Work out the finished part from the listing and answer in its coordinate system (mm). A direction names the side the tool comes from. Round coordinates to 2 decimals unless told otherwise and drop trailing zeros. Loops run counter-clockwise (first coordinate to the right, second up) from the corner with the lowest first, then second, coordinate; pieces in that order, holes last.
```python
from build123d import *

# Parameters (mm, degrees)
BOSS_EXTRUDE1_DEPTH = 4
SKETCH10_R          = 4
SKETCH10_R_2        = 2.5
SKETCH10_W          = 20
SKETCH10_H          = 5
BOSS_EXTRUDE5_DEPTH = 5
SKETCH11_W          = 3
SKETCH11_H          = 50
SKETCH11_W_2        = 40
SKETCH11_H_2        = 3
BOSS_EXTRUDE6_DEPTH = 4
SKETCH12_R          = 2.5
CUT_EXTRUDE5_DEPTH  = 4
BOSS_EXTRUDE7_START = 2
SKETCH13_R          = 4
SKETCH13_R_2        = 2.5
BOSS_EXTRUDE7_DEPTH = 2
SKETCH14_R          = 2
CUT_EXTRUDE6_DEPTH  = 15
SKETCH15_R          = 3.5
CUT_EXTRUDE8_DEPTH  = 2
FILLET1_R           = 5


with BuildPart() as part:
    # Sketch1 → Boss-Extrude1 (new body)
    with BuildSketch(Plane(origin=(0, 0, 0), x_dir=(1, 0, 0), z_dir=(0, 1, 0))):
        Polygon((-68, 48), (-88, 28), (-88, -48), (88, -48), (88, 28), (68, 48), align=None)
    extrude(amount=BOSS_EXTRUDE1_DEPTH)

    # Sketch10 → Boss-Extrude5 (add)
    # profile 1 of 5: a face of its own
    with BuildSketch(Plane(origin=(0, 4, 0), x_dir=(1, 0, 0), z_dir=(0, 1, 0))):
        with Locations(Location((36.5, -38, 0), (0, 0, 270))):
            Circle(SKETCH10_R)
        with Locations(Location((36.5, -38, 0), (0, 0, 270))):
            Circle(SKETCH10_R_2, mode=Mode.SUBTRACT)
    # profile 2 of 5: a face of its own
    with BuildSketch(Plane(origin=(0, 4, 0), x_dir=(1, 0, 0), z_dir=(0, 1, 0))):
        with Locations(Location((-37.5, -37.5, 0), (0, 0, 270))):
            Circle(SKETCH10_R)
        with Locations(Location((-37.5, -37.5, 0), (0, 0, 270))):
            Circle(SKETCH10_R_2, mode=Mode.SUBTRACT)
    # profile 3 of 5: a face of its own
    with BuildSketch(Plane(origin=(0, 4, 0), x_dir=(1, 0, 0), z_dir=(0, 1, 0))):
        with Locations(Location((-35, 23, 0), (0, 0, 270))):
            Circle(SKETCH10_R)
        with Locations(Location((-35, 23, 0), (0, 0, 270))):
            Circle(SKETCH10_R_2, mode=Mode.SUBTRACT)
    # profile 4 of 5: a face of its own
    with BuildSketch(Plane(origin=(0, 4, 0), x_dir=(1, 0, 0), z_dir=(0, 1, 0))):
        with Locations((62, 26)):
            Rectangle(SKETCH10_W, SKETCH10_H)
    # profile 5 of 5: a face of its own
    with BuildSketch(Plane(origin=(0, 4, 0), x_dir=(1, 0, 0), z_dir=(0, 1, 0))):
        Polygon((42, 23), (42, 15), (39, 15), (39, 26), (44, 26), (44, 23), align=None)
    extrude(amount=BOSS_EXTRUDE5_DEPTH)

    # Sketch11 → Boss-Extrude6 (add)
    with BuildSketch(Plane(origin=(0, 4, 0), x_dir=(1, 0, 0), z_dir=(0, 1, 0))):
        Polygon((25, 43.5), (25, 45), (-25, 45), (-25, 43.5), (-25, 42), (25, 42), align=None)
        Polygon((-82, 20), (-83.5, 20), (-85, 20), (-85, -30), (-82, -30), align=None)
        with Locations((83.5, -5)):
            Rectangle(SKETCH11_W, SKETCH11_H)
        with Locations((-45, -43.5)):
            Rectangle(SKETCH11_W_2, SKETCH11_H_2)
    extrude(amount=BOSS_EXTRUDE6_DEPTH)

    # Sketch12 → Cut-Extrude5 (cut)
    with BuildSketch(Plane(origin=(0, 4, 0), x_dir=(1, 0, 0), z_dir=(0, 1, 0))):
        with Locations(Location((-63, 0, 0), (0, 0, 270))):
            Circle(SKETCH12_R)
        with Locations(Location((-33, 0, 0), (0, 0, 270))):
            Circle(SKETCH12_R)
        with Locations(Location((-3, 0, 0), (0, 0, 270))):
            Circle(SKETCH12_R)
    extrude(amount=-CUT_EXTRUDE5_DEPTH, mode=Mode.SUBTRACT)

    # Sketch13 → Boss-Extrude7 (add)
    # profile 1 of 3: a face of its own
    with BuildSketch(Plane(origin=(0, 4, 0), x_dir=(1, 0, 0), z_dir=(0, 1, 0)).offset(BOSS_EXTRUDE7_START)):
        with Locations(Location((-63, 0, 0), (0, 0, 270))):
            Circle(SKETCH13_R)
        with Locations(Location((-63, 0, 0), (0, 0, 270))):
            Circle(SKETCH13_R_2, mode=Mode.SUBTRACT)
    # profile 2 of 3: a face of its own
    with BuildSketch(Plane(origin=(0, 4, 0), x_dir=(1, 0, 0), z_dir=(0, 1, 0)).offset(BOSS_EXTRUDE7_START)):
        with Locations(Location((-33, 0, 0), (0, 0, 270))):
            Circle(SKETCH13_R)
        with Locations(Location((-33, 0, 0), (0, 0, 270))):
            Circle(SKETCH13_R_2, mode=Mode.SUBTRACT)
    # profile 3 of 3: a face of its own
    with BuildSketch(Plane(origin=(0, 4, 0), x_dir=(1, 0, 0), z_dir=(0, 1, 0)).offset(BOSS_EXTRUDE7_START)):
        with Locations(Location((-3, 0, 0), (0, 0, 270))):
            Circle(SKETCH13_R)
        with Locations(Location((-3, 0, 0), (0, 0, 270))):
            Circle(SKETCH13_R_2, mode=Mode.SUBTRACT)
    extrude(amount=-BOSS_EXTRUDE7_DEPTH)

    # Sketch14 → Cut-Extrude6 (cut)
    with BuildSketch(Plane(origin=(0, 4, 0), x_dir=(1, 0, 0), z_dir=(0, 1, 0))):
        with Locations(Location((-65.928932188, 43, 0), (0, 0, 270))):
            Circle(SKETCH14_R)
        with Locations(Location((-83, 25.928932188, 0), (0, 0, 270))):
            Circle(SKETCH14_R)
        with Locations(Location((-83, -43, 0), (0, 0, 270))):
            Circle(SKETCH14_R)
        with Locations(Location((65.928932188, 43, 0), (0, 0, 270))):
            Circle(SKETCH14_R)
        with Locations(Location((83, 25.928932188, 0), (0, 0, 270))):
            Circle(SKETCH14_R)
        with Locations(Location((83, -43, 0), (0, 0, 270))):
            Circle(SKETCH14_R)
    extrude(amount=-CUT_EXTRUDE6_DEPTH, mode=Mode.SUBTRACT)

    # Sketch15 → Cut-Extrude8 (cut)
    with BuildSketch(Plane.XZ):
        with Locations(Location((-83, 43, 0), (0, 0, 270))):
            Circle(SKETCH15_R)
        with Locations(Location((-83, -25.928932188, 0), (0, 0, 270))):
            Circle(SKETCH15_R)
        with Locations(Location((-65.928932188, -43, 0), (0, 0, 270))):
            Circle(SKETCH15_R)
        with Locations(Location((65.928932188, -43, 0), (0, 0, 90))):
            Circle(SKETCH15_R)
        with Locations(Location((83, -25.928932188, 0), (0, 0, 90))):
            Circle(SKETCH15_R)
        with Locations(Location((83, 43, 0), (0, 0, 90))):
            Circle(SKETCH15_R)
    extrude(amount=-CUT_EXTRUDE8_DEPTH, mode=Mode.SUBTRACT)

    # Fillet1
    fillet1_edges = [part.edges().sort_by_distance(p)[0] for p in [
        (88, 2, 48),
        (-88, 2, 48),
        (-88, 2, -28),
        (-68, 2, -48),
        (68, 2, -48),
        (88, 2, -28),
    ]]
    fillet(fillet1_edges, radius=FILLET1_R)


solid = part.part
```
1. Find section C-C (x = 60). Write down the section's boundary in (y, z).
Answer key:
outline: (0, -48) - (4, -48) - (4, -28.5) - (9, -28.5) - (9, -23.5) - (4, -23.5) - (4, 48) - (0, 48) - close
2. Determine the mould class of faces 1 (the face through (-38.46, 6.46, 39.81)), 2 (the face through (62, 6, -23.5)), 3 (the face through (87.61, 2.03, -27.87)) for opening direction Z: +Z half, -Z half, draft (parallel to the pull), parting line (faces both ways), or undercut.
Answer key:
face 1: undercut
face 2: +Z half
face 3: -Z half
3. Which of the six approach directions +Z, -Z, +X, -X, +Y, -Y give full straight-line access (tool end or side, diameter ignored) to faces 4 (the face through (67, 2, -41)), 5 (the face through (72, 6, -26)), 6 (the face through (41, 6, -26))?
Answer key:
face 4: -Y
face 5: +Z, -Z, +X, +Y
face 6: -Z, +Y
4. Find section D-D (z = 0). Give the number of separate pieces and of enclosed holes in the cut face, then the cut area to 3 significant figures.
Answer key:
separate pieces: 4
enclosed holes: 0
area: 686 mm2
5. Find section A-A (x = -3). Write down the section's boundary in (y, z), then the cut area to 3 significant figures.
Answer key:
outline: (0, -48) - (4, -48) - (4, -45) - (8, -45) - (8, -42) - (4, -42) - (4, -4) - (6, -4) - (6, -2.5) - (0, -2.5) - close; (0, 2.5) - (6, 2.5) - (6, 4) - (4, 4) - (4, 48) - (0, 48) - close
area: 382 mm2
6. Find section B-B (z = -17). Write down the section's boundary in (x, y), then the cut area to 3 significant figures.
Answer key:
outline: (-88, 0) - (88, 0) - (88, 4) - (85, 4) - (85, 8) - (82, 8) - (82, 4) - (42, 4) - (42, 9) - (39, 9) - (39, 4) - (-82, 4) - (-82, 8) - (-85, 8) - (-85, 4) - (-88, 4) - close
area: 743 mm2
7. Consider probe 1 along X at (y, z) = (2.8, 43); probe 2 along X at (y, z) = (1.5, 0); probe 3 along X at (y, z) = (6.75, 2). Determine where each line is inside the solid, lowest interval first.
Answer key:
probe 1: x = -88 to -85, -81 to 81, 85 to 88
probe 2: x = -88 to -65.5, -60.5 to -35.5, -30.5 to -5.5, -0.5 to 88
probe 3: x = -85 to -82, 82 to 85
8. Given pin 1 (6.5 mm diameter, centred on x = 83, z = -25.93, fed in from +Y); pin 2 (3.5 mm diameter, centred on x = -65.93, z = -43, fed in from -Y); pin 3 (0.9 mm diameter, centred on y = 5.5, z = -43.5, fed in from +X); pin 4 (0.9 mm diameter, centred on x = -40.5, z = 44, fed in from +Y), each flat-ended and moving along its own axis, determine where each tip first touches the part or whether it passes through.
Answer key:
pin 1: stops at y = 4
pin 2: passes through
pin 3: stops at x = 25
pin 4: stops at y = 8
